Check sheet for the modelled part. Datum: model origin and axes. Units: mm. A direction names the side the tool comes from. Round coordinates to 2 decimals unless told otherwise and drop trailing zeros. Loops run counter-clockwise (first coordinate to the right, second up) from the corner with the lowest first, then second, coordinate; pieces in that order, holes last. Notation, with made-up numbers: (79, -0.75) - (90, -0.75) arc R19 ccw to (90, 27.25) - close; hole circle Ø4 at (-40, 12). An arc over 180 degrees is marked (long way). Answer in a Markdown table with one row per item. Add a question column.
(1) Access from +Z, -Z, +X, -X, +Y, -Y to the whole of each face (thin tool, end or side, straight path). Record for faces 5 (the flat face through (1, 0, -1.6)), 6 (the flat face through (0, 0, 0)), 7 (the flat face through (2.028, -6.936, 10.454)).
(2) Gauge pin test, flat ends, axial feed: pin 1 (0.7 mm diameter, centred on x = 0.5, z = -1, fed in from +Y); pin 2 (0.8 mm diameter, centred on x = 1.5, z = 0, fed in from -Y); pin 3 (1 mm diameter, centred on x = 1.5, y = -1, fed in from +Z). Record the tip position at first contact, or that the pin passes through.
(3) Mould release check, pull along Z, two halves, no side actions. Record for faces 1 (the cylindrical face through (2, -9.7, 13.6)), 2 (the cylindrical face through (2.028, -5.899, 15.662)), 3 (the flat face through (2.5, -1, 0)), 4 (the flat face through (4, -3, 6)): +Z half, -Z half, draft (parallel to the pull), parting line (faces both ways), or undercut.
(4) Cross-section at D-D on y = 2.25. Enter the section's corners in (x, z).
(5) Cross-section at B-B on x = 1. Count the separate pieces of the cut face and the enclosed holes in it, then the cut area to 3 significant figures.
(6) Cross-section at C-C on z = 0. Enter the section's corners in (x, y), then the cut area to 3 significant figures.
(7) Thickness scan on line 1 along Y through (x, z) = (0.7, 0); line 2 along Y through (x, z) = (2.4, -1.5); line 3 along Z through (x, y) = (1.9, 0.25). Record the ranges inside material, lowest first.
from build123d import *

# Parameters (mm, degrees)
SKETCH5_R           = 4
BOSS_EXTRUDE2_DEPTH = 4
BOSS_EXTRUDE3_DEPTH = 4
SKETCH7_R           = 2.6
CUT_EXTRUDE3_DEPTH  = 2.5
BOSS_EXTRUDE4_DEPTH = 2.5
FILLET1_R           = 0.3
CUT_EXTRUDE4_REACH  = 22.452
FILLET2_R           = 3


with BuildPart() as part:
    # Sketch5 → Boss-Extrude2 (new body)
    with BuildSketch(Plane(origin=(0, 0, 0), x_dir=(0, 0, -1), z_dir=(1, 0, 0))):
        Circle(SKETCH5_R)
    extrude(amount=BOSS_EXTRUDE2_DEPTH)

    # Sketch6 → Boss-Extrude3 (add)
    with BuildSketch(Plane(origin=(0, 0, 0), x_dir=(0, 0, -1), z_dir=(1, 0, 0))):
        Polygon((-1.408414688, 2.648842779), (1.408414688, -2.648842779), (-14.043168187, -10.864595127), (-16.859997563, -5.56690957), align=None)
    extrude(amount=BOSS_EXTRUDE3_DEPTH)

    # Sketch7 → Cut-Extrude3 (cut)
    with BuildSketch(Plane.ZY):
        Circle(SKETCH7_R)
    extrude(amount=-CUT_EXTRUDE3_DEPTH, mode=Mode.SUBTRACT)

    # Sketch8 → Boss-Extrude4 (add)
    with BuildSketch(Plane.ZY.offset(-2.5)):
        Polygon((1.6, -0.75), (-1.6, -0.75), (-1.6, 0.75), (-0.65, 0.75), (-0.65, 1.25), (0.65, 1.25), (0.65, 0.75), (1.6, 0.75), align=None)
    extrude(amount=BOSS_EXTRUDE4_DEPTH)

    # Fillet1
    fillet1_edges = [part.edges().sort_by_distance(p)[0] for p in [
        (1.25, -0.75, 1.6),
        (1.25, 0.75, 1.6),
        (1.25, 0.75, -1.6),
        (1.25, -0.75, -1.6),
    ]]
    fillet(fillet1_edges, radius=FILLET1_R)

    # Sketch10 → Cut-Extrude4 (cut, up to next)
    with BuildSketch(Plane(origin=(4, 0, 0), x_dir=(0, 0, -1), z_dir=(1, 0, 0)), mode=Mode.PRIVATE) as cut_extrude4_sk1:
        with BuildLine():
            Line((-8.923549544, -6.139086946), (-12.02808746, -7.755207093))
            ThreePointArc((-12.02808746, -7.755207093), (-13.815193727, -7.191734651), (-13.251721285, -5.404628385))
            Line((-13.251721285, -5.404628385), (-10.147183369, -3.788508238))
            ThreePointArc((-10.147183369, -3.788508238), (-8.360077103, -4.35198068), (-8.923549544, -6.139086946))
        make_face()
    cut_extrude4_tool1 = extrude(cut_extrude4_sk1.sketch, amount=-CUT_EXTRUDE4_REACH, mode=Mode.PRIVATE) & part.part
    add(cut_extrude4_tool1.solids().sort_by_distance((4, -5.771858, 11.087635))[0], mode=Mode.SUBTRACT)

    # Fillet2
    fillet2_edges = [part.edges().sort_by_distance(p)[0] for p in [
        (2, -10.864595127, 14.043168187),
        (2, -5.56690957, 16.859997563),
    ]]
    fillet(fillet2_edges, radius=FILLET2_R - 0.0001)  # a hair under: the kernel refuses the full size


solid = part.part
Answers:
| question | item | result |
|---|---|---|
| 1 | face 5 | -X |
| 1 | face 6 | +Z, -Z, -X, +Y, -Y |
| 1 | face 7 | +X, -X |
| 2 | pin 1 | stops at y = 3.95 |
| 2 | pin 2 | stops at y = -4 |
| 2 | pin 3 | stops at z = 9.21 |
| 3 | face 1 | parting line |
| 3 | face 2 | +Z half |
| 3 | face 3 | undercut |
| 3 | face 4 | draft |
| 4 | outline | (0, -3.31) - (4, -3.31) - (4, 3.31) - (0, 3.31) - (0, 1.3) - (2.5, 1.3) - (2.5, -1.3) - (0, -1.3) - close |
| 5 | separate pieces | 2 |
| 5 | enclosed holes | 2 |
| 5 | area | 99.2 mm^2 |
| 6 | outline | (0, -4) - (4, -4) - (4, 4) - (0, 4) - (0, 2.6) - (2.5, 2.6) - (2.5, 1.25) - (0, 1.25) - (0, -0.75) - (2.5, -0.75) - (2.5, -2.6) - (0, -2.6) - close |
| 6 | area | 24.0 mm^2 |
| 7 | line 1 | y = -4 to -2.6, -0.75 to 1.25, 2.6 to 4 |
| 7 | line 2 | y = -3.71 to -2.12, -0.67 to 0.67, 2.12 to 3.71 |
| 7 | line 3 | z = -3.99 to -2.59, -1.6 to 1.6, 2.59 to 5.92 |
